Input: dimensioned drawing with shaded views. Units: mm. Origin: part minimum x, y, z. A direction names the side the tool comes from. Round coordinates to 2 decimals unless told otherwise and drop trailing zeros. Loops run counter-clockwise (first coordinate to the right, second up) from the corner with the lowest first, then second, coordinate; pieces in that order, holes last.
Item 1: Section query A-A on x = 16. Return loops of the section in (y, z).
Item 2: Section query C-C on y = 77. Return loops of the section in (x, z) (1 decimal).
Item 3: First-contact query: P1, Ø3, axis at x = 24.5, y = 84.5, coming from the -Z side; P2, Ø4, axis at x = 47.5, y = 41, coming from the +Z side; P3, Ø10, axis at y = 87, z = 14, coming from the -X side; P4, Ø1.5, axis at x = 43.5, y = 119.5, coming from the +Z side (1 decimal). Flat tips, straight axial feed; report the tip coordinate or a pass-through.
Item 4: Access query for the marked faces 1 and 2. Directions: +Z, -Z, +X, -X, +Y, -Y. A direction counts if a zero-diameter tool reaches every point of the face in a straight line with its end or side. Return the directions, or none.
Item 5: Pull-direction query (Y, two-part tool) for the marked faces 3, 4 and 5; classes: released by +Y, released by -Y, zero draft, split by the parting line, or undercut.
Item 6: Ray query, L1, parallel to Z at x = 18.5, y = 41 (1 decimal); L2, parallel to Z at x = 41, y = 104.5 (1 decimal); L3, parallel to X at y = 8, z = 57.5 (1 decimal). Return the intervals inside material, ascending.
Item 7: Section query B-B on z = 79.5. Return loops of the section in (x, y) (1 decimal).
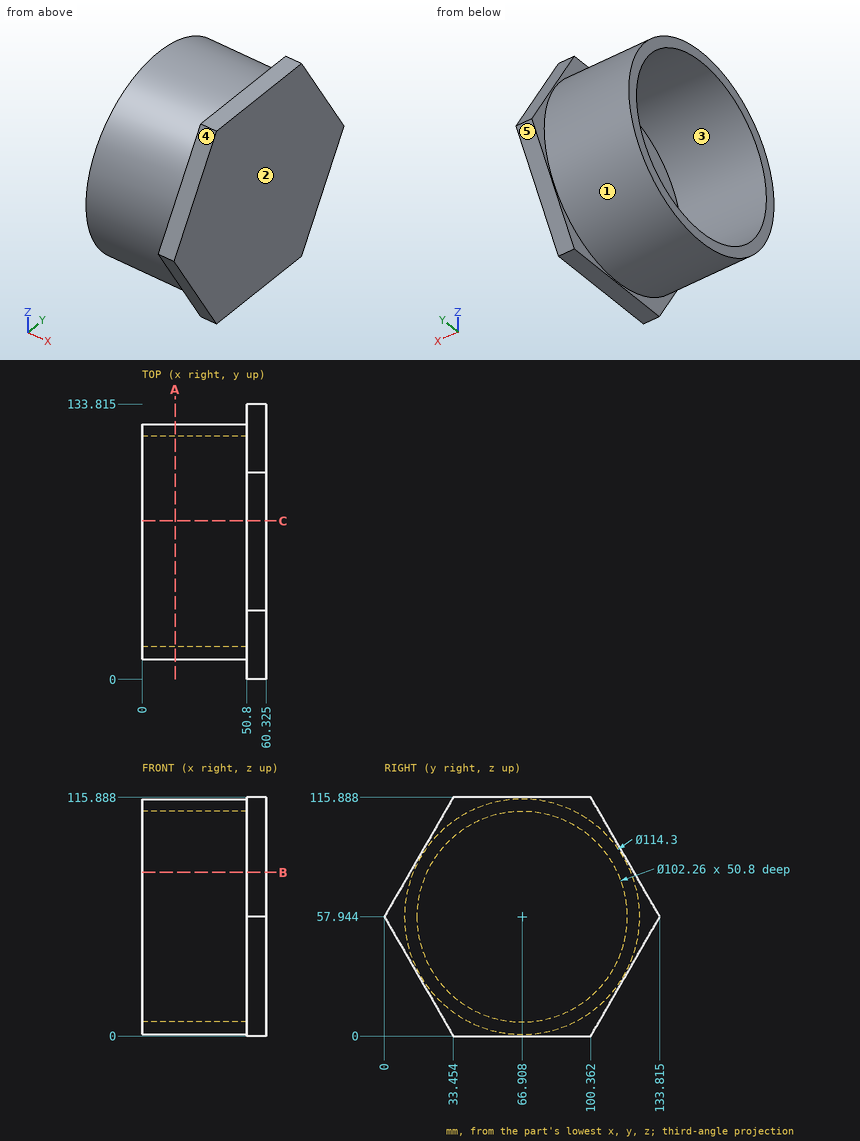
Data:
1. outline: circle Ø114.3 at (66.91, 57.94); hole circle Ø102.26 at (66.91, 57.94)
2. outline: (0, 1.7) - (50.8, 1.7) - (50.8, 0) - (60.3, 0) - (60.3, 115.9) - (50.8, 115.9) - (50.8, 114.2) - (0, 114.2) - (0, 108.1) - (50.8, 108.1) - (50.8, 7.8) - (0, 7.8) - close
3. P1: stops at z = 3.11
3. P2: stops at z = 109.85
3. P3: stops at x = 0
3. P4: stops at z = 82
4. face 1: -X
4. face 2: +Z, -Z, +X, +Y, -Y
5. face 3: undercut
5. face 4: released by -Y
5. face 5: released by +Y
6. L1: z = 7 to 13.9, 102 to 108.9
6. L2: z = 14.9 to 23.3, 92.6 to 101
6. L3: x = 50.8 to 60.3
7. outline: (0, 14) - (50.8, 14) - (50.8, 12.4) - (60.3, 12.4) - (60.3, 121.4) - (50.8, 121.4) - (50.8, 119.8) - (0, 119.8) - (0, 113.3) - (50.8, 113.3) - (50.8, 20.5) - (0, 20.5) - close
